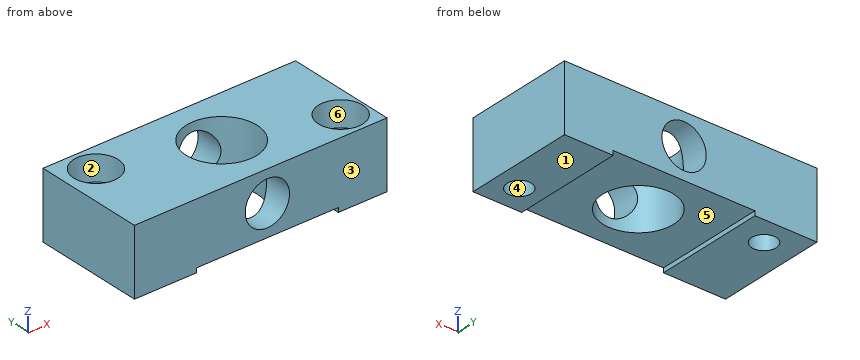
```python
from build123d import *

# Parameters (mm, degrees)
SKETCH1_R           = 5
BOSS_EXTRUDE2_DEPTH = 25
SKETCH3_R           = 2.75
SKETCH3_R_2         = 8
CUT_EXTRUDE1_DEPTH  = 16
SKETCH4_R           = 5
CUT_EXTRUDE2_DEPTH  = 5.7


with BuildPart() as part:
    # Sketch1 → Boss-Extrude2 (new body)
    with BuildSketch(Plane(origin=(0, 0, 0), x_dir=(1, 0, 0), z_dir=(0, 1, 0))):
        Polygon((-14.5, 7.5), (-14.5, 6.5), (17.5, 6.5), (17.5, 7.5), (28.5, 7.5), (28.5, -7.5), (-28.5, -7.5), (-28.5, 7.5), align=None)
        with Locations((1.5, -0.5)):
            Circle(SKETCH1_R, mode=Mode.SUBTRACT)
    extrude(amount=BOSS_EXTRUDE2_DEPTH)

    # Sketch3 → Cut-Extrude1 (cut, through all)
    with BuildSketch(Plane.XY.offset(7.5)):
        with Locations((-21.5, 19)):
            Circle(SKETCH3_R)
        with Locations((1.5, 12.5)):
            Circle(SKETCH3_R_2)
        with Locations((23, 6)):
            Circle(SKETCH3_R)
    extrude(amount=-CUT_EXTRUDE1_DEPTH, mode=Mode.SUBTRACT)

    # Sketch4 → Cut-Extrude2 (cut)
    with BuildSketch(Plane.XY.offset(7.5)):
        with Locations((-21.5, 19)):
            Circle(SKETCH4_R)
        with Locations((23, 6)):
            Circle(SKETCH4_R)
    extrude(amount=-CUT_EXTRUDE2_DEPTH, mode=Mode.SUBTRACT)


solid = part.part
```
Build history of the part. All positions in model axes, mm. Face numbers are marked on the shaded views. A direction names the side the tool comes from. Coordinates: 2 decimals unless noted, no trailing zeros. Order: outer loops, then holes, each group sorted by start corner. A loop starts at its lowest first (then second) coordinate and runs counter-clockwise, first axis right, second up.
Item 1: Mould opens along Y. For the marked faces 1, 2 and 3 say: released by +Y, released by -Y, zero draft, split by the parting line, or undercut.
Filled in:
face 1: zero draft
face 2: undercut
face 3: released by -Y
Item 2: Saw through at A-A on z = -5.5. List the corners of the cut face in (x, y).
Filled in:
outline: (-28.5, 0) - (28.5, 0) - (28.5, 25) - (-28.5, 25) - close; hole circle Ø5.5 at (-21.5, 19); hole circle Ø16 at (1.5, 12.5); hole circle Ø5.5 at (23, 6)
Item 3: Saw through at C-C on y = 12.5. List the corners of the cut face in (x, z), then the cut area to 3 significant figures.
Filled in:
outline: (-28.5, -7.5) - (-14.5, -7.5) - (-14.5, -6.5) - (-6.5, -6.5) - (-6.5, 7.5) - (-28.5, 7.5) - close; (9.5, -6.5) - (17.5, -6.5) - (17.5, -7.5) - (28.5, -7.5) - (28.5, 7.5) - (9.5, 7.5) - close
area: 599 mm2
Item 4: Saw through at B-B on x = 1.5. List the corners of the cut face in (y, z), then the cut area to 3 significant figures.
Filled in:
outline: (0, -6.5) - (4.5, -6.5) - (4.5, -4.5) - (0, -4.5) - close; (0, 5.5) - (4.5, 5.5) - (4.5, 7.5) - (0, 7.5) - close; (20.5, -6.5) - (25, -6.5) - (25, -4.5) - (20.5, -4.5) - close; (20.5, 5.5) - (25, 5.5) - (25, 7.5) - (20.5, 7.5) - close
area: 36.0 mm2
Item 5: Drill centre lines: L1, parallel to Y at x = -21.5, z = 5.95; L2, parallel to Z at x = 1.5, y = 22.5; L3, parallel to X at y = 21.5, z = 0.5. Where is each one in solid material? Low to high.
Filled in:
L1: y = 0 to 14, 24 to 25
L2: z = -6.5 to -4.5, 5.5 to 7.5
L3: x = -28.5 to -22.65, -20.35 to -3.5, 6.5 to 28.5
Item 6: Drop a flat-ended pin along its axis: pin 1 Ø12.5 at (x, y) = (4.5, 12) entering from -Z. Give the stop position or say it passes through.
Filled in:
pin 1: stops at z = -6.5
Item 7: Tool access for the marked faces 4, 5 and 6: list every direction of +Z, -Z, +X, -X, +Y, -Y with a clear straight run to the whole face (end or side of a thin tool).
Filled in:
face 4: +Z, -Z
face 5: -Z, +Y, -Y
face 6: +Z
Item 8: Saw through at D-D on x = 23. List the corners of the cut face in (y, z).
Filled in:
outline: (0, -7.5) - (3.25, -7.5) - (3.25, 1.8) - (1, 1.8) - (1, 7.5) - (0, 7.5) - close; (8.75, -7.5) - (25, -7.5) - (25, 7.5) - (11, 7.5) - (11, 1.8) - (8.75, 1.8) - close
